```python
from build123d import *

# Parameters (mm, degrees)
F0_R     = 3.5
F1_DEPTH = 7.85
F2_R     = 3.5
F2_R_2   = 2
F3_DEPTH = 8


with BuildPart() as f1:
    # F0 (on Top) → F1 (new body)
    with BuildSketch(Plane.XY):
        Circle(F0_R)
        with BuildLine():
            ThreePointArc((1.875, 1.801215), (2.411949, 0.970824), (2.6, 0))
            ThreePointArc((2.6, 0), (2.411949, -0.970824), (1.875, -1.801215))
            ThreePointArc((1.875, -1.801215), (0, -2.6), (-1.875, -1.801215))
            ThreePointArc((-1.875, -1.801215), (-2.6, 0), (-1.875, 1.801215))
            ThreePointArc((-1.875, 1.801215), (0, 2.6), (1.875, 1.801215))
        make_face(mode=Mode.SUBTRACT)
        with BuildLine():
            ThreePointArc((1.875, -1.801215), (2.411949, -0.970824), (2.6, 0))
            ThreePointArc((2.6, 0), (2.411949, 0.970824), (1.875, 1.801215))
            Line((1.875, 1.801215), (1.875, -1.801215))
        make_face()
        with BuildLine():
            Line((-1.875, -1.801215), (-1.875, 1.801215))
            ThreePointArc((-1.875, 1.801215), (-2.6, 0), (-1.875, -1.801215))
        make_face()
    extrude(amount=F1_DEPTH)

    # F2 (on face) → F3 (join)
    with BuildSketch(Plane.XY.offset(7.85)):
        Circle(F2_R)
        Circle(F2_R_2, mode=Mode.SUBTRACT)
    extrude(amount=F3_DEPTH)


solid = f1.part
```
CAD build for the part. Positions are in the model's coordinates, mm. A direction names the side the tool comes from. Round coordinates to 2 decimals unless told otherwise and drop trailing zeros. Order: outer loops, then holes, each group sorted by start corner. A loop starts at its lowest first (then second) coordinate and runs counter-clockwise, first axis right, second up.
Q1. Slice it at C-C (x = 0). Write the cut outline in (y, z), and give its area (3 significant figures).
Q2. Slice it at D-D (x = -3). Write the cut outline in (y, z), and give its area (3 significant figures).
Q3. Drop flat-ended pins along their axis: pin 1 (2 mm diameter, centred on x = 0.5, y = 1, fed in from -Z); pin 2 (3 mm diameter, centred on y = -2.5, z = 2, fed in from -X); pin 3 (3 mm diameter, centred on x = 0, y = 0, fed in from -Z); pin 4 (4 mm diameter, centred on x = 2.5, z = 5.5, fed in from -Y). Give the stop position or say it passes through.
Q4. Which spindle directions (+Z, -Z, +X, -X, +Y, -Y) get a long thin tool onto all of the face, cutting with end or side? Do faces 5 (the cylindrical face through (0, -2, 12)), 6 (the flat face through (1.875, 0, 4)), 7 (the flat face through (2.3, 0, 0)). Say none if no direction does.
Q5. Wall check: L1, parallel to Y at x = 0, z = 11.5; L2, parallel to X at y = -0.75, z = 5.5 (3 decimals); L3, parallel to Y at x = -1.5, z = 2.25. Give the ranges that are in metal, low to high.
Q6. Slice it at A-A (y = 0). Write the cut outline in (x, z) (3 decimals), and give its area (3 significant figures).
Q7. Slice it at B-B (z = 5.25). Write the cut outline in (x, y) (3 decimals), and give its area (3 significant figures).
Q8. Two-plate mould, pull along Y, no slides. Class faces 1 (the flat face through (0, -2.3, 7.85)), 2 (the flat face through (2, -2, 15.85)), 3 (the flat face through (-1.875, 0, 4)), 4 (the cylindrical face through (3.233, -1.341, 7.814)): pulls with the +Y half, pulls with the -Y half, needs draft (parallel to the pull), parting line crosses it, or undercut.
Results below:
1. outline: (-3.5, 0) - (-2.6, 0) - (-2.6, 7.85) - (-2, 7.85) - (-2, 15.85) - (-3.5, 15.85) - close; (2, 7.85) - (2.6, 7.85) - (2.6, 0) - (3.5, 0) - (3.5, 15.85) - (2, 15.85) - close
1. area: 38.1 mm2
2. outline: (-1.8, 0) - (1.8, 0) - (1.8, 15.85) - (-1.8, 15.85) - close
2. area: 57.1 mm2
3. pin 1: stops at z = 7.85
3. pin 2: stops at x = -3.35
3. pin 3: passes through
3. pin 4: stops at y = -3.46
4. face 5: +Z
4. face 6: -Z
4. face 7: -Z, +X, -X, +Y, -Y
5. L1: y = -3.5 to -2, 2 to 3.5
5. L2: x = -3.419 to -1.875, 1.875 to 3.419
5. L3: y = -3.16 to -2.12, 2.12 to 3.16
6. outline: (-3.5, 0) - (-1.875, 0) - (-1.875, 7.85) - (-2, 7.85) - (-2, 15.85) - (-3.5, 15.85) - close; (1.875, 0) - (3.5, 0) - (3.5, 15.85) - (2, 15.85) - (2, 7.85) - (1.875, 7.85) - close
6. area: 49.5 mm2
7. outline: circle Ø7 at (0, 0); hole (-1.875, -1.801) arc R2.6 ccw to (1.875, -1.801) - (1.875, 1.801) arc R2.6 ccw to (-1.875, 1.801) - close
7. area: 20.8 mm2
8. face 1: undercut
8. face 2: needs draft
8. face 3: undercut
8. face 4: parting line crosses it
